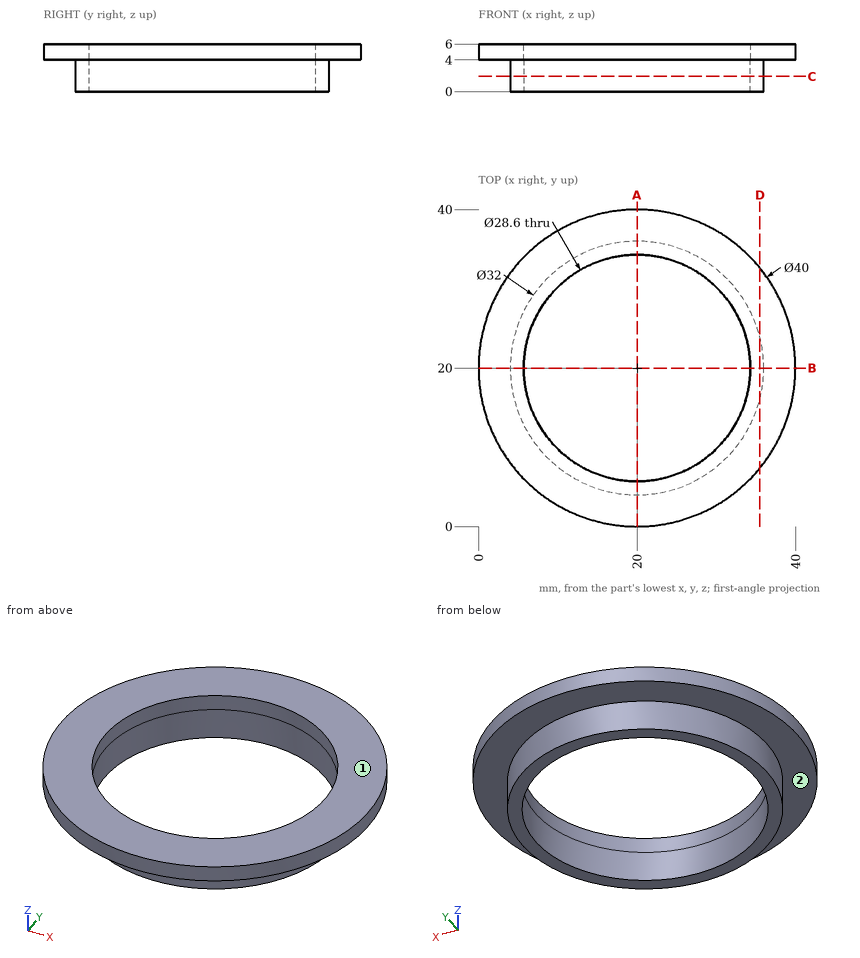
Geometry: see drawing. Coordinates: mm, zero at the bounding-box minimum. A direction names the side the tool comes from. Coordinates: 2 decimals unless noted, no trailing zeros. Loops run counter-clockwise (first coordinate to the right, second up) from the corner with the lowest first, then second, coordinate; pieces in that order, holes last. Notation, with made-up numbers: (72.25, 40) - (82.25, 40) arc R16 cw to (82.25, 58) - close; hole circle Ø11 at (-4, -38.75). An arc over 180 degrees is marked (long way). Put each result on its own line as item: value. Start each with the question number.
Q1. Line query: line 1 (X direction, y = 19.5, z = 0.7); line 2 (Y direction, x = 20, z = 4.7); line 3 (Y direction, x = 20, z = 1.8). Output: solid intervals per line, ascending.
Q2. Pin query (flat end, axial travel): pin 1 Ø1.5 at (x, z) = (22, 2.5) entering from -Y; pin 2 Ø3 at (y, z) = (11, 3.5) entering from -X; pin 3 Ø1 at (y, z) = (28.5, 2.5) entering from +X. Return the tip coordinate at first contact, or that it passes through.
Q3. Cut plane A-A, the plane x = 20. Return loops of the section in (y, z), and give its area (3 significant figures).
Q4. Set-up query: the marked faces 1 and 2. Return all of +Z, -Z, +X, -X, +Y, -Y with unobstructed straight access to the full face (end or side cutting, diameter ignored); none if empty.
Q5. Cut plane D-D, the plane x = 35.5. Return loops of the section in (y, z), and give its area (3 significant figures).
Q6. Cut plane C-C, the plane z = 1.9. Return loops of the section in (x, y).
Filled sheet:
1. line 1: 4.01 to 5.71, 34.29 to 35.99
1. line 2: 0 to 5.7, 34.3 to 40
1. line 3: 4 to 5.7, 34.3 to 36
2. pin 1: y = 4.05
2. pin 2: x = 1.49
2. pin 3: x = 33.86
3. outline: (0, 4) - (4, 4) - (4, 0) - (5.7, 0) - (5.7, 6) - (0, 6) - close; (34.3, 0) - (36, 0) - (36, 4) - (40, 4) - (40, 6) - (34.3, 6) - close
3. area: 36.4 mm²
4. face 1: +Z, +X, -X, +Y, -Y
4. face 2: -Z
5. outline: (7.36, 4) - (16.03, 4) - (16.03, 0) - (23.97, 0) - (23.97, 4) - (32.64, 4) - (32.64, 6) - (7.36, 6) - close
5. area: 82.3 mm²
6. outline: circle Ø32 at (20, 20); hole circle Ø28.6 at (20, 20)
